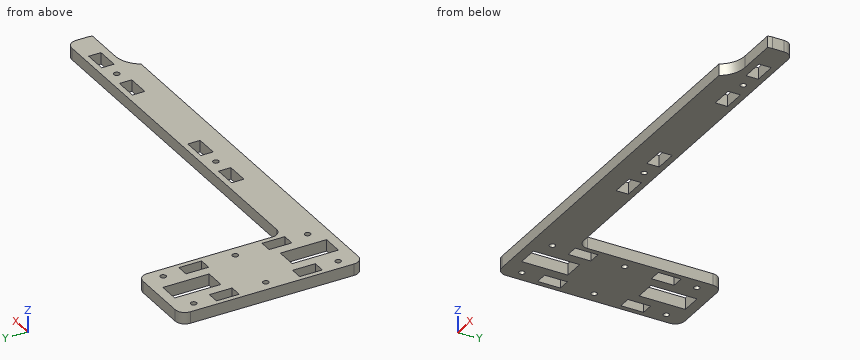
Autodesk Inventor part; units mm, degrees
ref_plane "YZ Plane" through (0, 0, 0) normal (1, 0, 0) x (0, 1, 0)
ref_plane "XZ Plane" through (0, 0, 0) normal (0, 1, 0) x (-1, 0, 0)
ref_plane "XY Plane" through (0, 0, 0) normal (0, 0, 1) x (1, 0, 0)
sketch "Sketch1" plane through (0, 0, 0) normal (0, 0, 1) x (1, 0, 0)
  line L0 (196.0836, -19.606) -> (216.6625, -19.606)
  arc A0 (216.6625, -19.606) -> (216.9836, -17.2233) centre (207.9836, -17.2233) ccw
  line L1 (216.9836, -17.2233) -> (216.9836, -11.2233)
  arc A1 (216.9836, -11.2233) -> (211.9836, -6.2233) centre (211.9836, -11.2233) ccw
  line L2 (211.9836, -6.2233) -> (26.9836, -6.2233)
  arc A2 (21.9836, -1.2233) -> (26.9836, -6.2233) centre (26.9836, -1.2233) ccw
  line L3 (21.9836, -1.2233) -> (21.9836, 63.7767)
  arc A3 (21.9836, 63.7767) -> (16.9836, 68.7767) centre (16.9836, 63.7767) ccw
  line L4 (16.9836, 68.7767) -> (-12.0164, 68.7767)
  arc A4 (-12.0164, 68.7767) -> (-17.0164, 63.7767) centre (-12.0164, 63.7767) ccw
  line L5 (-17.0164, 63.7767) -> (-17.0164, -21.2233)
  arc A5 (-17.0164, -21.2233) -> (-12.0164, -26.2233) centre (-12.0164, -21.2233) ccw
  line L6 (-12.0164, -26.2233) -> (184.2764, -26.2233)
  arc A6 (196.0836, -19.606) -> (184.2764, -26.2233) centre (196.0836, -33.4483) ccw
  circle A7 centre (-11.3164, 21.2767) radius 1.5
  circle A8 centre (16.2836, 21.2767) radius 1.5
  circle A9 centre (16.2836, -16.2233) radius 1.5
  circle A10 centre (-11.3164, -16.2233) radius 1.5
  circle A11 centre (92.5836, -12.4233) radius 1.5
  circle A12 centre (182.1836, -12.4233) radius 1.5
  circle A13 centre (-11.3164, 58.7767) radius 1.5
  circle A14 centre (16.2836, 58.7767) radius 1.5
  line L7 (13.0836, 36.9767) -> (13.0836, 48.7767)
  line L8 (13.0836, 48.7767) -> (19.4836, 48.7767)
  line L9 (19.4836, 48.7767) -> (19.4836, 36.9767)
  line L10 (19.4836, 36.9767) -> (13.0836, 36.9767)
  line L11 (-8.1164, 48.7767) -> (-8.1164, 36.9767)
  line L12 (-8.1164, 36.9767) -> (-14.5164, 36.9767)
  line L13 (-14.5164, 36.9767) -> (-14.5164, 48.7767)
  line L14 (-14.5164, 48.7767) -> (-8.1164, 48.7767)
  line L15 (13.0836, -6.2233) -> (13.0836, 5.5767)
  line L16 (13.0836, 5.5767) -> (19.4836, 5.5767)
  line L17 (19.4836, 5.5767) -> (19.4836, -6.2233)
  line L18 (19.4836, -6.2233) -> (13.0836, -6.2233)
  line L19 (201.9836, -9.2233) -> (201.9836, -15.6233)
  line L20 (201.9836, -15.6233) -> (190.1836, -15.6233)
  line L21 (190.1836, -15.6233) -> (190.1836, -9.2233)
  line L22 (190.1836, -9.2233) -> (201.9836, -9.2233)
  line L23 (174.1836, -9.2233) -> (174.1836, -15.6233)
  line L24 (174.1836, -15.6233) -> (162.3836, -15.6233)
  line L25 (162.3836, -15.6233) -> (162.3836, -9.2233)
  line L26 (162.3836, -9.2233) -> (174.1836, -9.2233)
  line L27 (112.3836, -9.2233) -> (112.3836, -15.6233)
  line L28 (112.3836, -15.6233) -> (100.5836, -15.6233)
  line L29 (100.5836, -15.6233) -> (100.5836, -9.2233)
  line L30 (100.5836, -9.2233) -> (112.3836, -9.2233)
  line L31 (84.5836, -9.2233) -> (84.5836, -15.6233)
  line L32 (84.5836, -15.6233) -> (72.7836, -15.6233)
  line L33 (72.7836, -15.6233) -> (72.7836, -9.2233)
  line L34 (72.7836, -9.2233) -> (84.5836, -9.2233)
  line L35 (-8.1164, 5.5767) -> (-8.1164, -6.2233)
  line L36 (-8.1164, -6.2233) -> (-14.5164, -6.2233)
  line L37 (-14.5164, -6.2233) -> (-14.5164, 5.5767)
  line L38 (-14.5164, 5.5767) -> (-8.1164, 5.5767)
  line L39 (7.8336, 63.7767) -> (7.8336, 39.7767)
  line L40 (7.8336, 39.7767) -> (-2.8664, 39.7767)
  line L41 (-2.8664, 39.7767) -> (-2.8664, 63.7767)
  line L42 (-2.8664, 63.7767) -> (7.8336, 63.7767)
  line L43 (7.8336, 2.7767) -> (7.8336, -21.2233)
  line L44 (7.8336, -21.2233) -> (-2.8664, -21.2233)
  line L45 (-2.8664, -21.2233) -> (-2.8664, 2.7767)
  line L46 (-2.8664, 2.7767) -> (7.8336, 2.7767)
  point P0 (0, 0)
  point P1 (0, 0)
extrude "Extrusion1" add sketch "Sketch1" along normal blind 6
properties part number "zCar_a"
Read the model definition and answer for the solid it produces. Units are mm, in the model's axes. Coordinates: 2 decimals unless noted, no trailing zeros. Loops run counter-clockwise (first coordinate to the right, second up) from the corner with the lowest first, then second, coordinate; pieces in that order, holes last. Notation, with made-up numbers: (29.25, 84.25) -> (47.25, 84.25) arc R13 cw to (47.25, 97.25) -> close; hole circle Ø9 at (-30, -11.75). An arc over 180 degrees is marked (long way). Write item = value, one per line. Start each with the question number.
1) Given P1, Ø2.5, axis at x = 182.18, y = -12.42, coming from the +Z side; P2, Ø1.5, axis at y = 40.5, z = 1, coming from the +X side, each flat-ended and moving along its own axis, determine where each tip first touches the part or whether it passes through.
2) Find the intervals of material crossed by L1, parallel to X at y = 4, z = 5.1; L2, parallel to X at y = 42, z = 0.55; L3, parallel to Y at x = 166, z = 0.4, in increasing order. Write a range as from..to.
3) The part is cut by section B-B, the plane x = 121. Determine the outline of the cut face in (y, z), plus the area to 3 significant figures.
4) The part is cut by section C-C, the plane z = 1.25. State how many separate pieces and enclosed holes the cut face has, plus the area to 3 significant figures.
5) The part is cut by section D-D, the plane y = 27. Determine the outline of the cut face in (x, z).
6) The part is cut by section A-A, the plane y = 44.5. Determine the outline of the cut face in (x, z).
Result:
q1.P1 = through
q1.P2 = 21.98
q2.L1 = -17.02..-14.52, -8.12..13.08, 19.48..21.98
q2.L2 = -17.02..-14.52, -8.12..-2.87, 7.83..13.08, 19.48..21.98
q2.L3 = -26.22..-15.62, -9.22..-6.22
q3.outline = (-26.22, 0) -> (-6.22, 0) -> (-6.22, 6) -> (-26.22, 6) -> close
q3.area = 120 mm²
q4.separate_pieces = 1
q4.enclosed_holes = 18
q4.area = 6,220 mm²
q5.outline = (-17.02, 0) -> (21.98, 0) -> (21.98, 6) -> (-17.02, 6) -> close
q6.outline = (-17.02, 0) -> (-14.52, 0) -> (-14.52, 6) -> (-17.02, 6) -> close; (-8.12, 0) -> (-2.87, 0) -> (-2.87, 6) -> (-8.12, 6) -> close; (7.83, 0) -> (13.08, 0) -> (13.08, 6) -> (7.83, 6) -> close; (19.48, 0) -> (21.98, 0) -> (21.98, 6) -> (19.48, 6) -> close
